Geometry: see drawing. Coordinates: mm, zero at the bounding-box minimum. A direction names the side the tool comes from. Coordinates: 2 decimals unless noted, no trailing zeros. Order: outer loops, then holes, each group sorted by start corner. A loop starts at its lowest first (then second) coordinate and runs counter-clockwise, first axis right, second up.
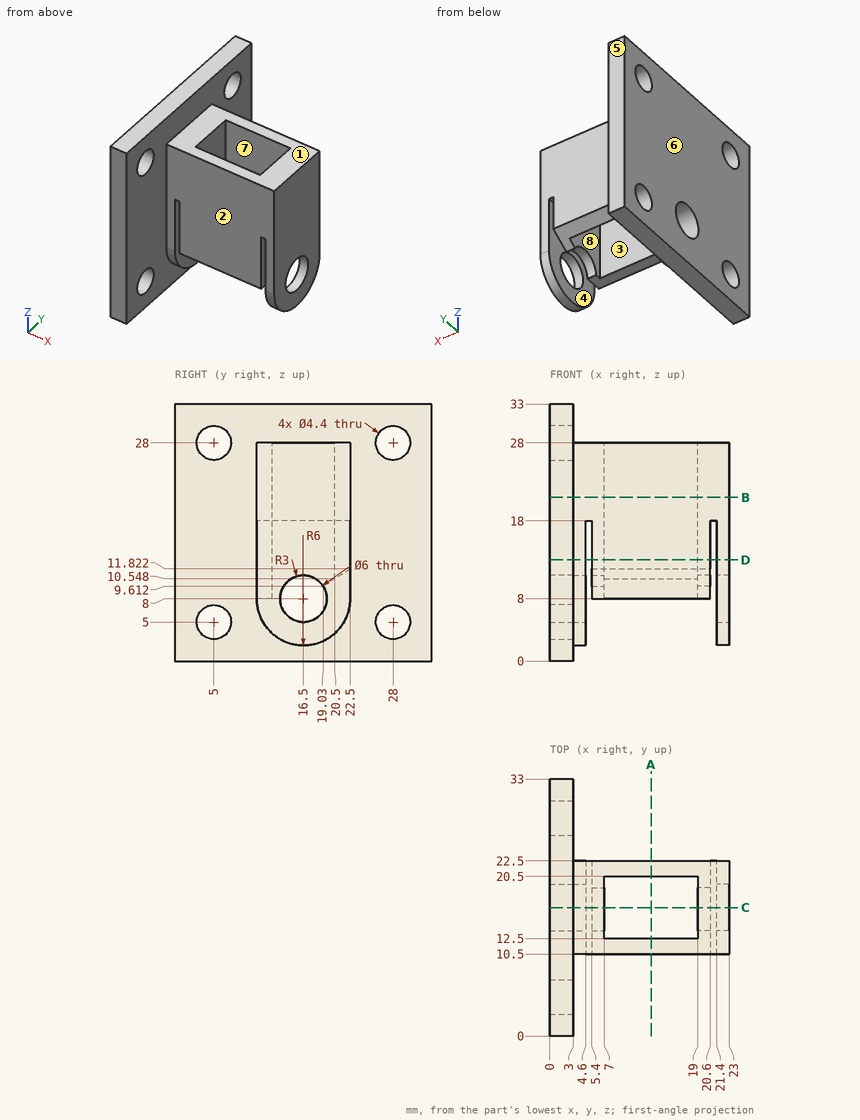
Q1. Pin query (flat end, axial travel): P1, Ø7, axis at y = 28, z = 5, coming from the +X side; P2, Ø3.5, axis at x = 15.5, z = 14, coming from the +Y side; P3, Ø9.5, axis at x = 16.5, y = 14.5, coming from the +Z side; P4, Ø6, axis at x = 11, y = 26.5, coming from the +Z side. Return the tip coordinate at first contact, or that it passes through.
Solutions:
P1: stops at x = 3
P2: stops at y = 22.5
P3: stops at z = 28
P4: passes through
Q2. Material intervals for line 1 along Y through (x, z) = (1.7, 28); line 2 along X through (y, z) = (11, 14); line 3 along X through (y, z) = (13.5, 3), sorted ascending.
Solutions:
line 1: y = 0 to 2.8, 7.2 to 25.8, 30.2 to 33
line 2: x = 0 to 4.6, 5.4 to 20.6, 21.4 to 23
line 3: x = 0 to 4.6, 21.4 to 23
Q3. Set-up query: the marked faces 1, 2, 3 and 4. Return all of +Z, -Z, +X, -X, +Y, -Y with unobstructed straight access to the full face (end or side cutting, diameter ignored); none if empty.
Solutions:
face 1: +Z, +X, +Y, -Y
face 2: +Z, -Z, +X, -Y
face 3: +Z, -Z
face 4: -Z, +Y, -Y
Q4. Section query A-A on x = 13. Output: boundary loops of the cut face in (y, z).
Solutions:
outline: (10.5, 8) - (12.5, 8) - (12.5, 28) - (10.5, 28) - close; (20.5, 10.55) - (22.5, 11.82) - (22.5, 28) - (20.5, 28) - close
Q5. Pull-direction query (X, two-part tool) for the marked faces 5, 6, 7 and 8; classes: pulls with the +X half, pulls with the -X half, needs draft (parallel to the pull), parting line crosses it, or undercut.
Solutions:
face 5: needs draft
face 6: pulls with the -X half
face 7: undercut
face 8: undercut
Q6. Section query D-D on z = 13. Output: boundary loops of the cut face in (x, y), plus the area to 3 significant figures.
Solutions:
outline: (0, 0) - (3, 0) - (3, 10.5) - (4.6, 10.5) - (4.6, 22.5) - (3, 22.5) - (3, 33) - (0, 33) - close; (5.4, 10.5) - (20.6, 10.5) - (20.6, 22.5) - (5.4, 22.5) - close; (21.4, 10.5) - (23, 10.5) - (23, 22.5) - (21.4, 22.5) - close; hole (7, 12.5) - (19, 12.5) - (19, 20.5) - (7, 20.5) - close
area: 224 mm2
Q7. Section query C-C on y = 16.5. Output: boundary loops of the cut face in (x, z).
Solutions:
outline: (0, 0) - (3, 0) - (3, 2) - (4.6, 2) - (4.6, 5) - (0, 5) - close; (0, 11) - (4.6, 11) - (4.6, 18) - (5.4, 18) - (5.4, 11) - (7, 11) - (7, 28) - (3, 28) - (3, 33) - (0, 33) - close; (19, 11) - (20.6, 11) - (20.6, 18) - (21.4, 18) - (21.4, 11) - (23, 11) - (23, 28) - (19, 28) - close; (21.4, 2) - (23, 2) - (23, 5) - (21.4, 5) - close
Q8. Section query B-B on z = 21. Output: boundary loops of the cut face in (x, y).
Solutions:
outline: (0, 0) - (3, 0) - (3, 10.5) - (23, 10.5) - (23, 22.5) - (3, 22.5) - (3, 33) - (0, 33) - close; hole (7, 12.5) - (19, 12.5) - (19, 20.5) - (7, 20.5) - close
